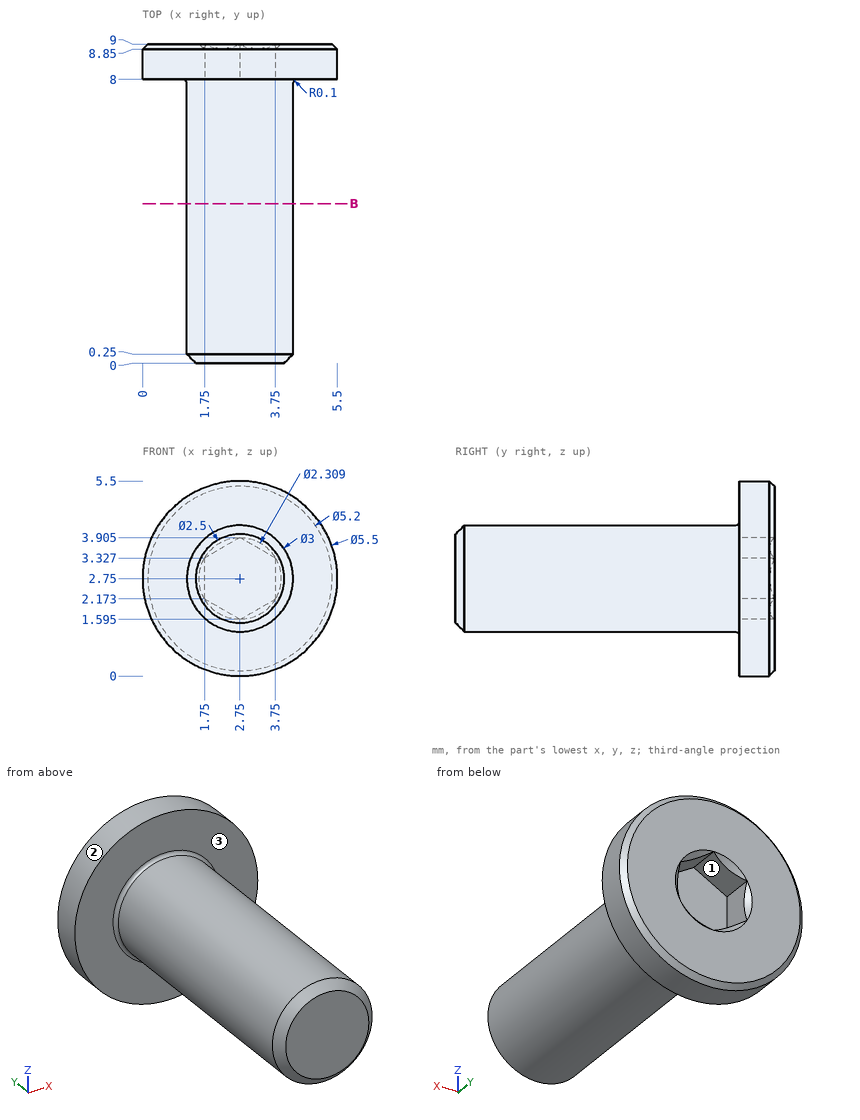
The figure shows three views and two pictorial views of one solid part (mm, origin at its lowest corner). Answer the questions. A direction names the side the tool comes from. Round coordinates to 2 decimals unless told otherwise and drop trailing zeros. Write each loop counter-clockwise with the first axis right and the second up, starting at its lowest first coordinate (ties: lowest second). Pieces come first, ordered by that corner, then holes. Notation, with made-up numbers: (13, 15.25) - (53, 15.25) arc R14 ccw to (53, 31.25) - close; hole circle Ø11 at (86, 26). An arc over 180 degrees is marked (long way). Answer in a Markdown table with one row per item. Add a question column.
1. Given pin 1 (1.5 mm diameter, centred on x = 4, y = 2, fed in from -Z) (1 decimal); pin 2 (0.5 mm diameter, centred on y = 8.5, z = 2.5, fed in from -X); pin 3 (1.5 mm diameter, centred on x = 4, y = 3.5, fed in from +Z) (1 decimal); pin 4 (3 mm diameter, centred on y = 4.5, z = 4.5, fed in from +X), each flat-ended and moving along its own axis, determine where each tip first touches the part or whether it passes through.
2. For the marked faces 1, 2 and 3, determine the directions among +Z, -Z, +X, -X, +Y, -Y from which every point of the face is accessible in a straight line to the end or side of a thin tool.
3. A cutting plane is placed at B-B, the plane y = 4.5. Determine the outline of the cut face in (x, z).
4. Find the intervals of material crossed by line 1 along Y through (x, z) = (1.1, 1.5); line 2 along Y through (x, z) = (3, 3.2); line 3 along X through (y, z) = (8.5, 1.4) (1 decimal), in increasing order. Write a range as from..to.
Worked out:
| question | item | result |
|---|---|---|
| 1 | pin 1 | z = 1.3 |
| 1 | pin 2 | x = 0 |
| 1 | pin 3 | z = 4.2 |
| 1 | pin 4 | x = 4.23 |
| 2 | face 1 | +Y |
| 2 | face 2 | +Y, -Y |
| 2 | face 3 | -Y |
| 3 | outline | circle Ø3 at (2.75, 2.75) |
| 4 | line 1 | 8..9 |
| 4 | line 2 | 0..8 |
| 4 | line 3 | 0.4..5.1 |
